from build123d import *

# Parameters (mm, degrees)
SKETCH1_W           = 900
SKETCH1_H           = 900
BOSS_EXTRUDE1_DEPTH = 600
SKETCH3_W           = 880
SKETCH3_H           = 100
CUT_EXTRUDE2_DEPTH  = 850


with BuildPart() as part:
    # Sketch1 → Boss-Extrude1 (new body)
    with BuildSketch(Plane(origin=(0, 0, 0), x_dir=(1, 0, 0), z_dir=(0, 1, 0))):
        Rectangle(SKETCH1_W, SKETCH1_H)
    extrude(amount=BOSS_EXTRUDE1_DEPTH)

    # Sketch3 → Cut-Extrude2 (cut)
    with BuildSketch(Plane(origin=(450, 0, 0), x_dir=(0, 0, -1), z_dir=(1, 0, 0))):
        with Locations((0, 60)):
            Rectangle(SKETCH3_W, SKETCH3_H)
        with Locations((0, 190)):
            Rectangle(SKETCH3_W, SKETCH3_H)
        with Locations((0, 320)):
            Rectangle(SKETCH3_W, SKETCH3_H)
        with Locations((0, 450)):
            Rectangle(SKETCH3_W, SKETCH3_H)
        with Locations((0, 580)):
            Rectangle(SKETCH3_W, SKETCH3_H)
    extrude(amount=-CUT_EXTRUDE2_DEPTH, mode=Mode.SUBTRACT)


solid = part.part
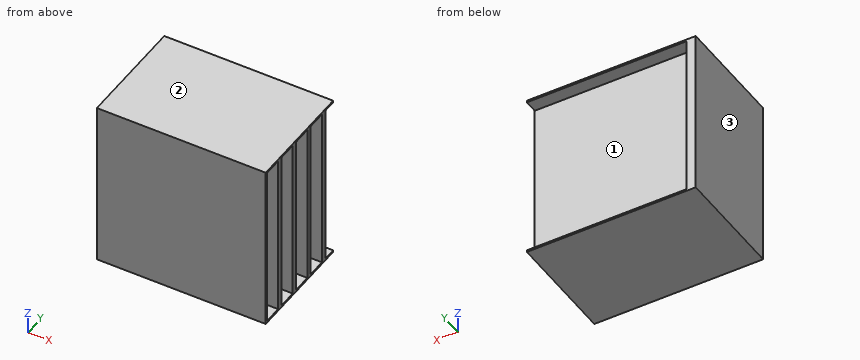
Can you work these out from the model? Positions are in its coordinate system, mm. Face numbers are marked on the shaded views. Give positions to 0.01 mm unless a question says otherwise; leave off trailing zeros. Order: outer loops, then holes, each group sorted by start corner. A loop starts at its lowest first (then second) coordinate and runs counter-clockwise, first axis right, second up. Notation, with made-up numbers: M 42,40 L 88,40 A26 cw 88,77 Z; hole C 33.5,33.25 d8. An arc over 180 degrees is marked long. One line per item, written item: value.
Item 1: If we section it at C-C on z = -221: Write out the boundary of the cut face in (x, y), and give its area (4 significant figures).
Verdict:
outline: M -450,0 L 450,0 L 450,10 L -400,10 L -400,110 L 450,110 L 450,140 L -400,140 L -400,240 L 450,240 L 450,270 L -400,270 L -400,370 L 450,370 L 450,400 L -400,400 L -400,500 L 450,500 L 450,530 L -400,530 L -400,600 L -450,600 Z
area: 140,500 mm2
Item 2: If we mould it in two halves opening along Z, with no side actions, what happens to the marked faces 1, 2 and 3? For each: pulls with the +Z half, pulls with the -Z half, needs draft (parallel to the pull), parting line crosses it, or undercut.
Verdict:
face 1: undercut
face 2: pulls with the +Z half
face 3: needs draft
Item 3: For pin 1 (2 mm diameter, centred on y = 160.5, z = 142.5, fed in from +X); pin 2 (5 mm diameter, centred on x = 196, z = -304.5, fed in from +Y), each with a flat end and sliding along its axis, tell me the tip position at first contact or that it passes through.
Verdict:
pin 1: x = -400
pin 2: y = 530
Item 4: If we section it at B-B on y = 560.5: Write out the boundary of the cut face in (x, z), and give its area (3 significant figures).
Verdict:
outline: M -450,-450 L 450,-450 L 450,-440 L -400,-440 L -400,440 L 450,440 L 450,450 L -450,450 Z
area: 62,000 mm2
Item 5: If we section it at A-A on x = 312.5: Write out the boundary of the cut face in (y, z).
Verdict:
outline: M 0,-450 L 600,-450 L 600,-440 L 530,-440 L 530,440 L 600,440 L 600,450 L 0,450 Z; hole M 10,-440 L 110,-440 L 110,440 L 10,440 Z; hole M 140,-440 L 240,-440 L 240,440 L 140,440 Z; hole M 270,-440 L 370,-440 L 370,440 L 270,440 Z; hole M 400,-440 L 500,-440 L 500,440 L 400,440 Z
Item 6: Please list where these lines run through material, in increasing order: line 1 (Y direction, x = 112, z = -107); line 2 (Z direction, x = 2, y = 143); line 3 (X direction, y = 107, z = -351).
Verdict:
line 1: 0 to 10, 110 to 140, 240 to 270, 370 to 400, 500 to 530
line 2: -450 to -440, 440 to 450
line 3: -450 to -400
